from build123d import *

# Parameters (mm, degrees)
BOSS_EXTRU_1_DEPTH           = 10
R_P_TITION_CIRCULAIRE2_COUNT = 7
ESQUISSE5_R                  = 4.5
BOSS_EXTRU_2_DEPTH           = 10


with BuildPart() as part:
    # Esquisse4 → Boss.-Extru.1 (new body)
    with BuildSketch(Plane.XY):
        with BuildLine():
            Line((0, 6.577848346), (0, 4.5))
            ThreePointArc((0, 4.5), (1.039097311, 4.378387463), (2.022031395, 4.020123013))
            Line((2.022031395, 4.020123013), (2.955692415, 5.876391002))
            ThreePointArc((2.955692415, 5.876391002), (3.02541978, 7.297456647), (2.538901994, 8.634464469))
            ThreePointArc((2.538901994, 8.634464469), (2.078194622, 8.756774927), (1.611657757, 8.854521968))
            ThreePointArc((1.611657757, 8.854521968), (0.576250392, 7.878703818), (0, 6.577848346))
        make_face()
    extrude(amount=BOSS_EXTRU_1_DEPTH)


with BuildPart() as r_p_tition_circulaire2_1:
    # R_p_tition circulaire2: pattern copy
    add(part.part.rotate(Axis((0, 0, 0), (0, 0, 1)), 1 * 360 / R_P_TITION_CIRCULAIRE2_COUNT))


with BuildPart() as r_p_tition_circulaire2_2:
    # R_p_tition circulaire2: pattern copy
    add(part.part.rotate(Axis((0, 0, 0), (0, 0, 1)), 2 * 360 / R_P_TITION_CIRCULAIRE2_COUNT))


with BuildPart() as r_p_tition_circulaire2_3:
    # R_p_tition circulaire2: pattern copy
    add(part.part.rotate(Axis((0, 0, 0), (0, 0, 1)), 3 * 360 / R_P_TITION_CIRCULAIRE2_COUNT))


with BuildPart() as r_p_tition_circulaire2_4:
    # R_p_tition circulaire2: pattern copy
    add(part.part.rotate(Axis((0, 0, 0), (0, 0, 1)), 4 * 360 / R_P_TITION_CIRCULAIRE2_COUNT))


with BuildPart() as r_p_tition_circulaire2_5:
    # R_p_tition circulaire2: pattern copy
    add(part.part.rotate(Axis((0, 0, 0), (0, 0, 1)), 5 * 360 / R_P_TITION_CIRCULAIRE2_COUNT))


with BuildPart() as r_p_tition_circulaire2_6:
    # R_p_tition circulaire2: pattern copy
    add(part.part.rotate(Axis((0, 0, 0), (0, 0, 1)), 6 * 360 / R_P_TITION_CIRCULAIRE2_COUNT))


with BuildPart() as part_1:
    add(part.part)

    add(r_p_tition_circulaire2_1.part)  # Boss.-Extru.2 merges R_p_tition circulaire2_1

    add(r_p_tition_circulaire2_2.part)  # Boss.-Extru.2 merges R_p_tition circulaire2_2

    add(r_p_tition_circulaire2_3.part)  # Boss.-Extru.2 merges R_p_tition circulaire2_3

    add(r_p_tition_circulaire2_4.part)  # Boss.-Extru.2 merges R_p_tition circulaire2_4

    add(r_p_tition_circulaire2_5.part)  # Boss.-Extru.2 merges R_p_tition circulaire2_5

    add(r_p_tition_circulaire2_6.part)  # Boss.-Extru.2 merges R_p_tition circulaire2_6
    # Esquisse5 → Boss.-Extru.2 (add)
    with BuildSketch(Plane.XY):
        Circle(ESQUISSE5_R)
    extrude(amount=BOSS_EXTRU_2_DEPTH)


solid = part_1.part
Can you work these out from the model? Positions are in its coordinate system, mm. A direction names the side the tool comes from. Give positions to 0.01 mm unless a question says otherwise; leave off trailing zeros. Order: outer loops, then holes, each group sorted by start corner. A loop starts at its lowest first (then second) coordinate and runs counter-clockwise, first axis right, second up. Notation, with made-up numbers: M -36.5,63.5 L -0.5,63.5 A33 cw -0.5,97.5 Z; hole C 27.5,22 d3. An arc over 180 degrees is marked long. Use one line per item in the form item = value.
Item 1: For faces 1 (the cylindrical face through (-3.96, -6.86, 4.93)), 2 (the cylindrical face through (7.566, -2.33, 4.93)), 3 (the cylindrical face through (-4.077, -1.905, 4.93)), which set-ups out of +Z, -Z, +X, -X, +Y, -Y let a thin tool reach every point of the face, with its end or its side?
Values follow:
face_1 = +Z, -Z, -Y
face_2 = +Z, -Z, +X
face_3 = +Z, -Z
Item 2: Thinking about a two-plate mould opening in X: for faces 4 (the cylindrical face through (-5.806, 5.382, 4.93)), 5 (the flat face through (4.34, 3.46, 4.93)), 6 (the cylindrical face through (3.03, 7.28, 4.93)), 7 (the flat face through (0, 0, 10)), which applies, pulls with the +X half, pulls with the -X half, needs draft (parallel to the pull), parting line crosses it, or undercut?
Values follow:
face_4 = pulls with the -X half
face_5 = undercut
face_6 = pulls with the +X half
face_7 = needs draft
Item 3: If I drill on line 1 along Y through (x, z) = (-4.75, 4.75); line 2 along Y through (x, z) = (-5, 7.75); line 3 along Y through (x, z) = (6.5, 3.75), over which ranges is the centre line in solid material (lowest first)? Write a range as [from, to].
Values follow:
line_1 = [-7.18, -3.66], [-1.08, 1.17], [3.79, 7.29]
line_2 = [-7.23, -3.85], [-1.14, 1.23], [3.99, 7.34]
line_3 = [-4.58, -1.51], [1.38, 4.46]
Item 4: If we section it at C-C, the plane x = -1: Write out the boundary of the cut face in (y, z), and give its area (3 significant figures).
Values follow:
outline = M -4.39,0 L 4.39,0 L 4.39,10 L -4.39,10 Z
area = 87.7 mm^2
Item 5: If we section it at A-A, the plane y = 5.25: Write out the boundary of the cut face in (x, z), and give its area (3 significant figures).
Values follow:
outline = M -5.77,0 L -2.42,0 L -2.42,10 L -5.77,10 Z; M 0,0 L 2.64,0 L 2.64,10 L 0,10 Z
area = 59.9 mm^2
Item 6: Will these pins go through, and if not, where does the flat tip stop? pin 1 Ø0.6 at (y, z) = (5.5, 3.5) entering from -X; pin 2 Ø3 at (y, z) = (-3, 3) entering from -X; pin 3 Ø5 at (x, z) = (-2.5, 8) entering from -Y.
Values follow:
pin_1 = -5.9
pin_2 = -5.56
pin_3 = -7.23
Item 7: If we section it at B-B, the plane x = 6: Write out the boundary of the cut face in (y, z).
Values follow:
outline = M -4.51,0 L -1.37,0 L -1.37,10 L -4.51,10 Z; M 1.26,0 L 4.39,0 L 4.39,10 L 1.26,10 Z
Item 8: If we section it at D-D, the plane y = -2: Write out the boundary of the cut face in (x, z).
Values follow:
outline = M -4.03,0 L 7.23,0 L 7.23,10 L -4.03,10 Z
